The drawing under review shows one solid part. Ordinate dimensions are in mm from its lowest x, y, z. A direction names the side the tool comes from. Round coordinates to 2 decimals unless told otherwise and drop trailing zeros. Write each loop counter-clockwise with the first axis right and the second up, starting at its lowest first coordinate (ties: lowest second). Pieces come first, ordered by that corner, then holes. Notation, with made-up numbers: (-39.5, 15.5) - (-30.5, 15.5) arc R27 ccw to (-30.5, 51.5) - close; hole circle Ø4 at (77.25, 79). An arc over 180 degrees is marked (long way). Answer in a Markdown table with one row per item. Add a question column.
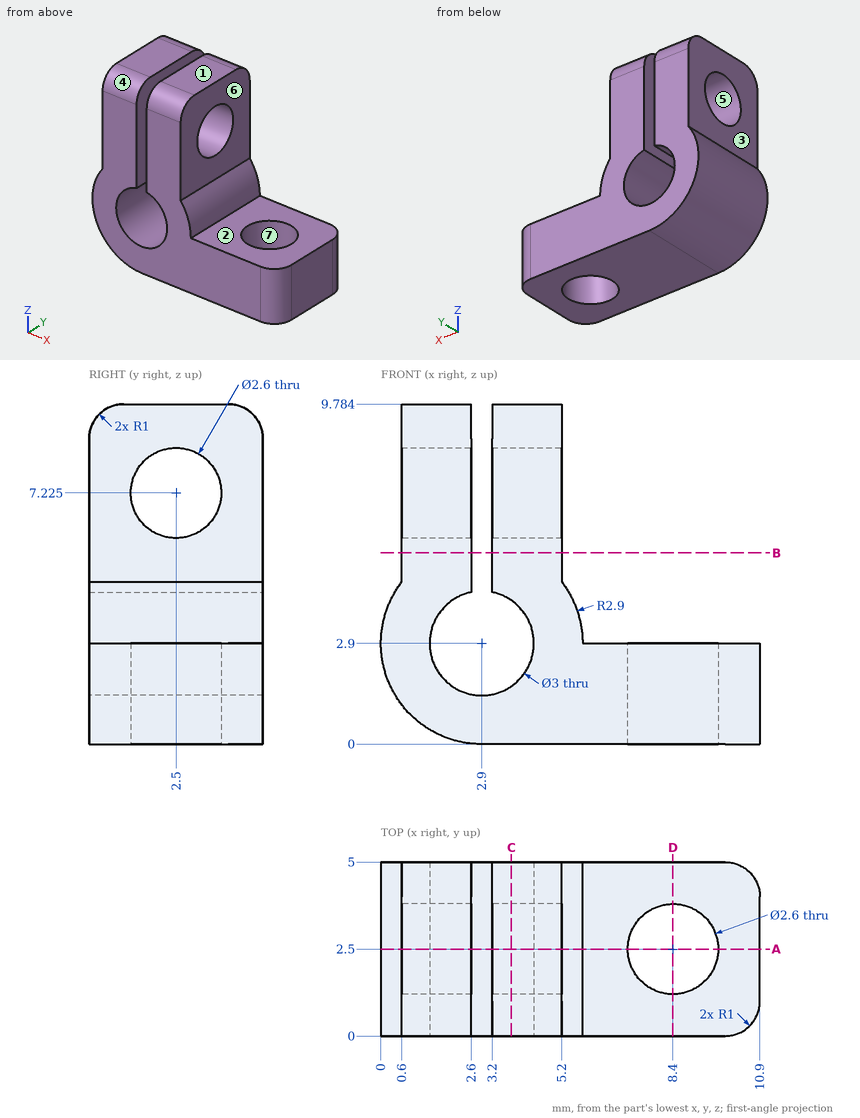
Q1. Add section B-B on z = 5.5. State the section outline as (x, y) points.
Q2. Tool access review of the marked faces 1, 2 and 3: name each direction out of +Z, -Z, +X, -X, +Y, -Y from which nothing blocks a thin tool from reaching the whole face with its end or side.
Q3. Insertion check: pin 1 Ø3 at (x, y) = (8.4, 2.5) entering from -Z; pin 2 Ø1.5 at (y, z) = (3.5, 7) entering from +X; pin 3 Ø2.5 at (y, z) = (1.5, 7) entering from -X; pin 4 Ø2.5 at (x, y) = (8.5, 3) entering from +Z. Each pin has a flat end and moves straight along its axis. Give the tip position at first contact, or say it passes through.
Q4. Add section A-A on y = 2.5. State the section outline as (x, z) points (1 decimal).
Q5. Add section D-D on x = 8.4. State the section outline as (y, z) points.
Q6. To check wall thickness, follow probe 1 along X at (y, z) = (1.3, 6); probe 2 along X at (y, z) = (1.4, 1.75) (1 decimal); probe 3 along Z at (x, y) = (2.5, 2.9) (1 decimal). State the ranges of each line that lie inside material, in increasing order.
Q7. Add section C-C on x = 3.75. State the section outline as (y, z) points (1 decimal).
Q8. Draft analysis for pull direction Y (two halves, no side actions). For the marked faces 4, 5, 6 and 7, state which applies: released by +Y, released by -Y, zero draft, split by the parting line, or undercut.
Answer sheet:
| question | item | result |
|---|---|---|
| 1 | outline | (0.6, 0) - (2.6, 0) - (2.6, 5) - (0.6, 5) - close; (3.2, 0) - (5.2, 0) - (5.2, 5) - (3.2, 5) - close |
| 2 | face 1 | +Z, +X, -X, +Y, -Y |
| 2 | face 2 | +Z, +X, +Y, -Y |
| 2 | face 3 | +Z, -X, +Y, -Y |
| 3 | pin 1 | stops at z = 0 |
| 3 | pin 2 | stops at x = 5.2 |
| 3 | pin 3 | stops at x = 0.6 |
| 3 | pin 4 | stops at z = 2.9 |
| 4 | outline | (0.6, 4.7) arc R2.9 ccw to (2.9, 0) - (7.1, 0) - (7.1, 2.9) - (5.8, 2.9) arc R2.9 ccw to (5.2, 4.7) - (5.2, 5.9) - (3.2, 5.9) - (3.2, 4.4) arc R1.5 cw (long way) to (2.6, 4.4) - (2.6, 5.9) - (0.6, 5.9) - close; (0.6, 8.5) - (2.6, 8.5) - (2.6, 9.8) - (0.6, 9.8) - close; (3.2, 8.5) - (5.2, 8.5) - (5.2, 9.8) - (3.2, 9.8) - close; (9.7, 0) - (10.9, 0) - (10.9, 2.9) - (9.7, 2.9) - close |
| 5 | outline | (0, 0) - (1.2, 0) - (1.2, 2.9) - (0, 2.9) - close; (3.8, 0) - (5, 0) - (5, 2.9) - (3.8, 2.9) - close |
| 6 | probe 1 | x = 0.6 to 2.6, 3.2 to 5.2 |
| 6 | probe 2 | x = 0.2 to 1.9, 3.9 to 7.7, 9.1 to 10.9 |
| 6 | probe 3 | z = 0 to 1.5, 4.3 to 6, 8.5 to 9.8 |
| 7 | outline | (0, 0) - (5, 0) - (5, 1.7) - (0, 1.7) - close; (0, 4.1) - (5, 4.1) - (5, 8.8) arc R1 ccw to (4, 9.8) - (1, 9.8) arc R1 ccw to (0, 8.8) - close; hole circle Ø2.6 at (2.5, 7.2) |
| 8 | face 4 | released by -Y |
| 8 | face 5 | undercut |
| 8 | face 6 | zero draft |
| 8 | face 7 | undercut |
